Build history of the part. All positions in model axes, mm. Face numbers are marked on the shaded views. A direction names the side the tool comes from. Give positions to 0.01 mm unless a question says otherwise; leave off trailing zeros. Order: outer loops, then holes, each group sorted by start corner. A loop starts at its lowest first (then second) coordinate and runs counter-clockwise, first axis right, second up. Notation, with made-up numbers: (-5.75, -29) - (21.25, -29) arc R26 cw to (21.25, -9) - close; hole circle Ø6 at (1, -25.5). An arc over 180 degrees is marked (long way). Write each question's results on one line, items separated by ' | '. Start each with the question number.
1) Cut at B-B on x = 0. List the corners of the cut face in (y, z).
2) Cut at C-C on z = -1. List the corners of the cut face in (x, y).
3) Tool access for the marked faces 1 and 2: list every direction of +Z, -Z, +X, -X, +Y, -Y with a clear straight run to the whole face (end or side of a thin tool).
4) Cut at D-D on z = 8.5. List the corners of the cut face in (x, y).
5) Drop flat-ended pins along their axis: pin 1 Ø1 at (y, z) = (-3.5, 2.5) entering from +X; pin 2 Ø3 at (y, z) = (0.5, 4.5) entering from +X; pin 3 Ø7 at (y, z) = (-20.5, 4.5) entering from +X; pin 4 Ø5 at (x, z) = (-0.5, 1) entering from +Y. Give the stop position or say it passes through.
6) Cut at A-A on y = 0. List the corners of the cut face in (x, z).
7) Drill centre lines: line 1 along Z through (x, y) = (-22.5, -13); line 2 along X through (y, z) = (3.5, 7.5); line 3 along Y through (x, z) = (-18, 9.25). Where is each one in solid material? Low to high. Write a range as from..to.
from build123d import *

# Parameters (mm, degrees)
F0_R     = 22.5
F1_DEPTH = 10
F2_R     = 27.5
F3_DEPTH = 3
F4_SIZE  = 0.4
F6_DEPTH = 25


with BuildPart() as f1:
    # F0 (on Top) → F1 (new body)
    with BuildSketch(Plane.XY):
        Circle(F0_R)
    extrude(amount=F1_DEPTH)

    # F2 (on face) → F3 (join)
    with BuildSketch(Plane(origin=(0, 0, 0), x_dir=(1, 0, 0), z_dir=(0, 0, -1))):
        Circle(F2_R)
    extrude(amount=F3_DEPTH)

    # F4
    f4_edges = [f1.edges().sort_by_distance(p)[0] for p in [
        (-27.5, 0, -3),
    ]]
    chamfer(f4_edges, length=F4_SIZE)

    # F5 (on face) → F6 (cut)
    with BuildSketch(Plane.XY.offset(10)):
        with BuildLine():
            Line((4, -27.207536), (4, -18.5))
            ThreePointArc((4, -18.5), (0, -14.5), (-4, -18.5))
            Line((-4, -18.5), (-4, -27.207536))
            ThreePointArc((-4, -27.207536), (0, -27.5), (4, -27.207536))
        make_face()
    extrude(amount=-F6_DEPTH, mode=Mode.SUBTRACT)


solid = f1.part
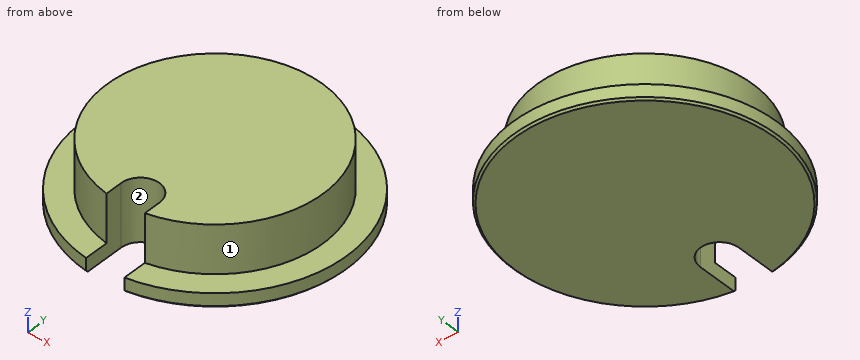
Results:
1) outline: (-14.5, -3) - (27.1, -3) - (27.5, -2.6) - (27.5, 0) - (22.5, 0) - (22.5, 10) - (-14.5, 10) - close
2) outline: (-4, -27.21) - (-4, -18.5) arc R4 cw to (4, -18.5) - (4, -27.21) arc R27.5 ccw (long way) to start
3) face 1: +Z | face 2: +Z, -Z, -Y
4) outline: (-4, -22.14) - (-4, -18.5) arc R4 cw to (4, -18.5) - (4, -22.14) arc R22.5 ccw (long way) to start
5) pin 1: x = 22.3 | pin 2: x = 22.5 | pin 3: x = 14.74 | pin 4: y = 27.5
6) outline: (-27.5, -2.6) - (-27.1, -3) - (27.1, -3) - (27.5, -2.6) - (27.5, 0) - (22.5, 0) - (22.5, 10) - (-22.5, 10) - (-22.5, 0) - (-27.5, 0) - close
7) line 1: -3..0 | line 2: -22.23..22.23 | line 3: -13.5..13.5
